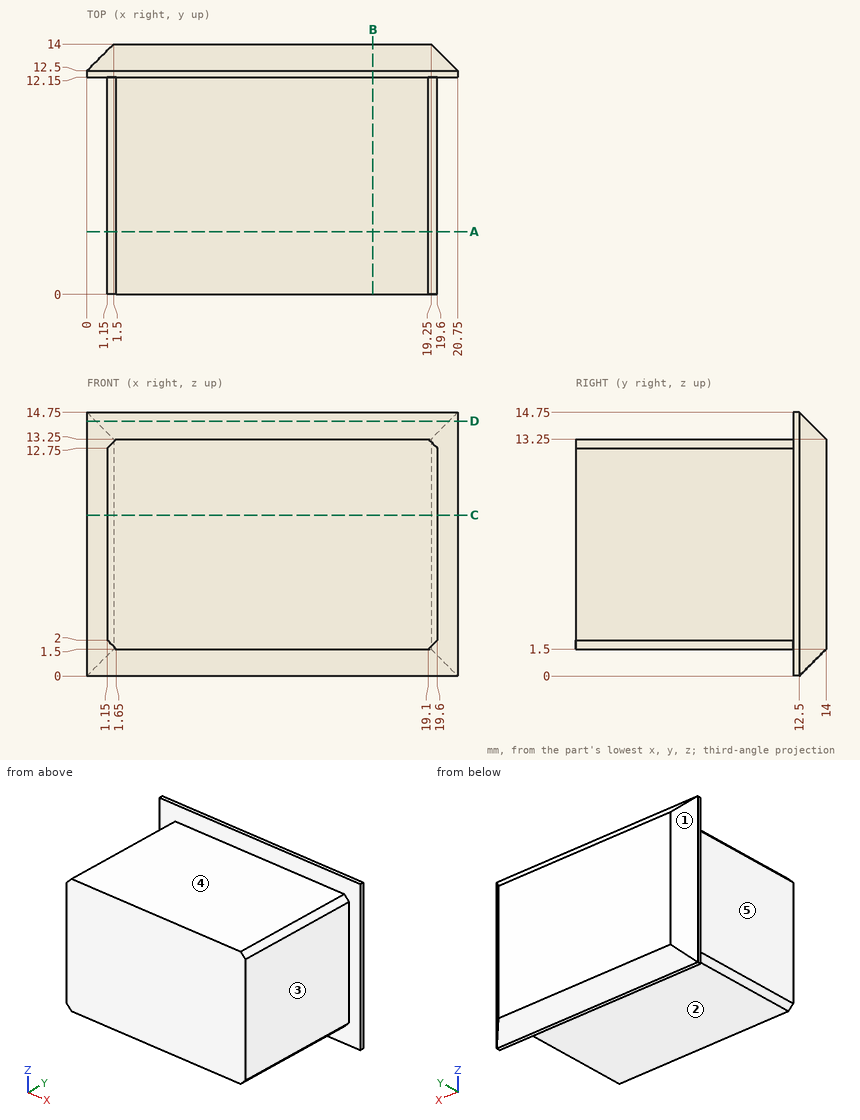
Geometry: see drawing. Coordinates: mm, zero at the bounding-box minimum. A direction names the side the tool comes from. Coordinates: 2 decimals unless noted, no trailing zeros. Loops run counter-clockwise (first coordinate to the right, second up) from the corner with the lowest first, then second, coordinate; pieces in that order, holes last.
Q1. Material intervals for line 1 (Z direction, x = 10.75, y = 6.75); line 2 (X direction, y = 5, z = 11.75); line 3 (Z direction, x = 12.5, y = 13), sorted ascending.
Q2. Contact query for flat-ended pins moving along their axis: pin 1 (4 mm diameter, centred on x = 11, y = 2, fed in from -Z); pin 2 (3 mm diameter, centred on x = 7.5, y = 9, fed in from +Z); pin 3 (5 mm diameter, centred on y = 9.5, z = 5.5, fed in from -X). Output: stop coordinate, or through.
Q3. Set-up query: the marked faces 1, 2, 3, 4 and 5. Return all of +Z, -Z, +X, -X, +Y, -Y with unobstructed straight access to the full face (end or side cutting, diameter ignored); none if empty.
Q4. Cut plane C-C (z = 9). Output: boundary loops of the cut face in (x, y).
Q5. Cut plane D-D (z = 14.25). Output: boundary loops of the cut face in (x, y).
Q6. Cut plane A-A (y = 3.5). Output: boundary loops of the cut face in (x, z).
Q7. Cut plane B-B (x = 16). Output: boundary loops of the cut face in (y, z).
Working result:
1. line 1: z = 1.5 to 13.25
1. line 2: x = 1.15 to 19.6
1. line 3: z = 0.5 to 14.25
2. pin 1: stops at z = 1.5
2. pin 2: stops at z = 13.25
2. pin 3: stops at x = 1.15
3. face 1: +Z, -Z, -X, +Y
3. face 2: -Z, +X, -X, -Y
3. face 3: +Z, -Z, +X, -Y
3. face 4: +Z, +X, -X, -Y
3. face 5: +Z, -Z, -X, -Y
4. outline: (0, 12.15) - (1.15, 12.15) - (1.15, 0) - (19.6, 0) - (19.6, 12.15) - (20.75, 12.15) - (20.75, 12.5) - (19.25, 14) - (1.5, 14) - (0, 12.5) - close
5. outline: (0, 12.15) - (20.75, 12.15) - (20.75, 12.5) - (20.25, 13) - (0.5, 13) - (0, 12.5) - close
6. outline: (1.15, 2) - (1.65, 1.5) - (19.1, 1.5) - (19.6, 2) - (19.6, 12.75) - (19.1, 13.25) - (1.65, 13.25) - (1.15, 12.75) - close
7. outline: (0, 1.5) - (12.15, 1.5) - (12.15, 0) - (12.5, 0) - (14, 1.5) - (14, 13.25) - (12.5, 14.75) - (12.15, 14.75) - (12.15, 13.25) - (0, 13.25) - close
